Part model, mm, in its own coordinate system. Face numbers are marked on the shaded views. A direction names the side the tool comes from. Round coordinates to 2 decimals unless told otherwise and drop trailing zeros. Write each loop counter-clockwise with the first axis right and the second up, starting at its lowest first coordinate (ties: lowest second). Pieces come first, ordered by that corner, then holes.
1) Pull direction Z, two halves, no side cores. Call the marked faces 3, 4 and 5: +Z half, -Z half, draft (parallel to the pull), parting line (faces both ways), or undercut.
2) Saw through at D-D on z = 136.5. Write the cut outline in (x, y).
3) Flat gauge pins, fed straight in: pin 1 (6 mm diameter, centred on x = -50, z = 20, fed in from -Y); pin 2 (10 mm diameter, centred on y = 24, z = 120.5, fed in from +X); pin 3 (6 mm diameter, centred on x = 55, y = -25, fed in from -Z); pin 4 (6 mm diameter, centred on x = 14, z = 117, fed in from -Y). Where does each tip first touch, or does it go through?
4) Drill centre lines: L1, parallel to Z at x = 8, y = -53.5; L2, parallel to Y at x = 0, z = 93; L3, parallel to Y at x = 0, z = 37. Where is each one in solid material? Low to high.
5) Saw through at C-C on z = 115.5. Write the cut outline in (x, y).
6) Which spindle directions (+Z, -Z, +X, -X, +Y, -Y) get a long thin tool onto all of the face, cutting with end or side? Do the marked faces 1 and 2. Say none if no direction does.
```python
from build123d import *

# Parameters (mm, degrees)
F0_R      = 54
F0_R_2    = 50
F1_DEPTH  = 150
F2_R      = 74
F2_R_2    = 54
F3_DEPTH  = 20
F4_R      = 74
F4_R_2    = 54
F5_DEPTH  = 20
F7_R      = 74
F7_R_2    = 54
F8_DEPTH  = 20
F10_R     = 74
F10_R_2   = 54
F11_DEPTH = 20


with BuildPart() as f1:
    # F0 (on Top) → F1 (new body)
    with BuildSketch(Plane.XY):
        Circle(F0_R)
        Circle(F0_R_2, mode=Mode.SUBTRACT)
    extrude(amount=F1_DEPTH)

    # F2 (on Top) → F3 (join)
    with BuildSketch(Plane.XY):
        Circle(F2_R)
        Circle(F2_R_2, mode=Mode.SUBTRACT)
    extrude(amount=F3_DEPTH)

    # F4 (on face) → F5 (join)
    with BuildSketch(Plane.XY.offset(150)):
        Circle(F4_R)
        Circle(F4_R_2, mode=Mode.SUBTRACT)
    extrude(amount=-F5_DEPTH)

    # F7 (on offset) → F8 (join)
    with BuildSketch(Plane(origin=(0, 0, 105), x_dir=(1, 0, 0), z_dir=(0, 0, -1))):
        Circle(F7_R)
        Circle(F7_R_2, mode=Mode.SUBTRACT)
    extrude(amount=F8_DEPTH)

    # F10 (on offset) → F11 (join)
    with BuildSketch(Plane(origin=(0, 0, 60), x_dir=(1, 0, 0), z_dir=(0, 0, -1))):
        Circle(F10_R)
        Circle(F10_R_2, mode=Mode.SUBTRACT)
    extrude(amount=F11_DEPTH)


solid = f1.part
```
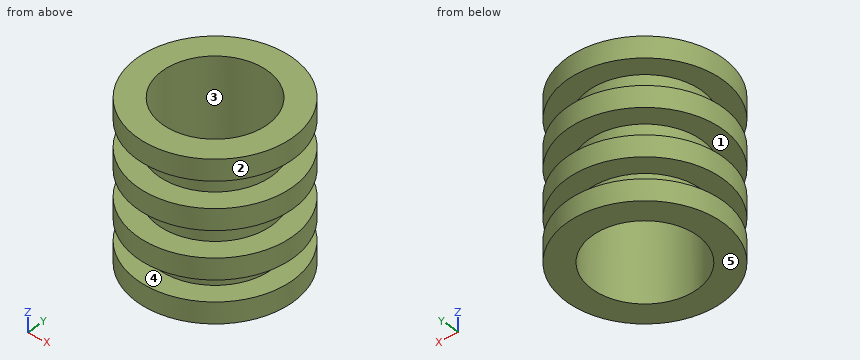
Completed:
1. face 3: draft
1. face 4: undercut
1. face 5: -Z half
2. outline: circle Ø148 at (0, 0); hole circle Ø100 at (0, 0)
3. pin 1: stops at y = -57.16
3. pin 2: stops at x = 50.55
3. pin 3: stops at z = 0
3. pin 4: stops at y = -52.87
4. L1: z = 0 to 20, 40 to 60, 85 to 105, 130 to 150
4. L2: y = -74 to -50, 50 to 74
4. L3: y = -54 to -50, 50 to 54
5. outline: circle Ø108 at (0, 0); hole circle Ø100 at (0, 0)
6. face 1: none
6. face 2: +Z, -Z
